Job drawing, mm, ordinate dimensions from the low corner. One solid piece. Coordinates: 2 decimals unless noted, no trailing zeros. Loops run counter-clockwise (first coordinate to the right, second up) from the corner with the lowest first, then second, coordinate; pieces in that order, holes last. Notation, with made-up numbers: (81.5, 1.25) - (132.5, 1.25) arc R10 ccw to (132.5, 10.25) - close; hole circle Ø6 at (-23.75, 8.25). An arc over 180 degrees is marked (long way). Use a Markdown table: item, result. Add a question column.
1. Band-saw the part on A-A, the plane y = 8.25. Give the cut face in (x, z).
2. Wall check: probe 1 along X at (y, z) = (1.75, 35); probe 2 along X at (y, z) = (4, 35.5) (1 decimal); probe 3 along Z at (x, y) = (50, 6). Give the ranges that are in metal, low to high. Write a range as [from, to].
3. Pull direction X, two halves, no side cores. Call the marked faces 1, 2, 3 and 4: pulls with the +X half, pulls with the -X half, needs draft (parallel to the pull), parting line crosses it, or undercut.
4. Band-saw the part on B-B, the plane x = 46.5. Give the cut face in (y, z), plus the area to 3 significant figures.
5. Band-saw the part on D-D, the plane y = 1.75. Give the cut face in (x, z).
6. Drop flat-ended pins along their axis: pin 1 (1 mm diameter, centred on x = 10.5, z = 52.5, fed in from -Y); pin 2 (6 mm diameter, centred on x = 11.5, y = 6.5, fed in from -Z); pin 3 (1 mm diameter, centred on y = 8, z = 56, fed in from +X). Give the stop position or say it passes through.
7. Band-saw the part on C-C, the plane z = 39. Give the cut face in (x, y) (1 decimal), plus the area to 3 significant figures.
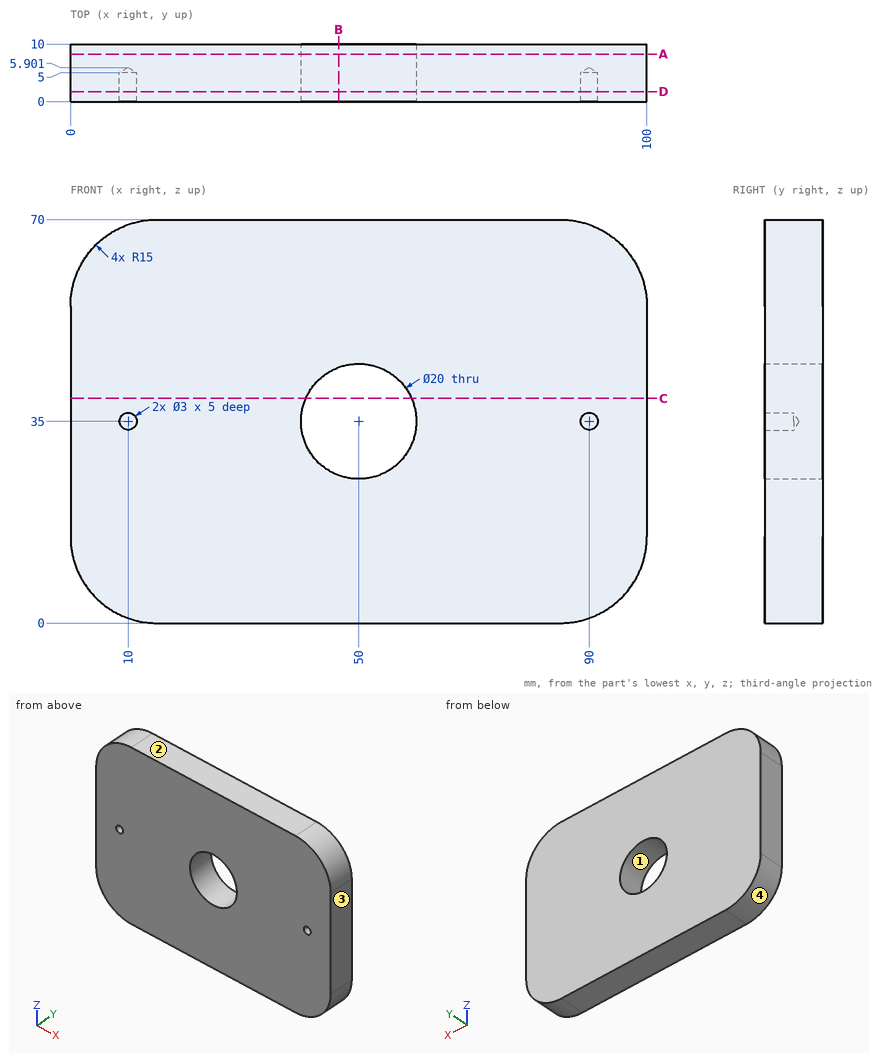
Geometry check:
| question | item | result |
|---|---|---|
| 1 | outline | (0, 15) arc R15 ccw to (15, 0) - (85, 0) arc R15 ccw to (100, 15) - (100, 55) arc R15 ccw to (85, 70) - (15, 70) arc R15 ccw to (0, 55) - close; hole circle Ø20 at (50, 35) |
| 2 | probe 1 | x = [0, 8.5], [11.5, 40], [60, 88.5], [91.5, 100] |
| 2 | probe 2 | x = [0, 8.6], [11.4, 40], [60, 88.6], [91.4, 100] |
| 2 | probe 3 | z = [0, 25], [45, 70] |
| 3 | face 1 | undercut |
| 3 | face 2 | needs draft |
| 3 | face 3 | pulls with the +X half |
| 3 | face 4 | pulls with the -X half |
| 4 | outline | (0, 0) - (10, 0) - (10, 25.63) - (0, 25.63) - close; (0, 44.37) - (10, 44.37) - (10, 70) - (0, 70) - close |
| 4 | area | 513 mm^2 |
| 5 | outline | (0, 15) arc R15 ccw to (15, 0) - (85, 0) arc R15 ccw to (100, 15) - (100, 55) arc R15 ccw to (85, 70) - (15, 70) arc R15 ccw to (0, 55) - close; hole circle Ø3 at (10, 35); hole circle Ø20 at (50, 35); hole circle Ø3 at (90, 35) |
| 6 | pin 1 | stops at y = 0 |
| 6 | pin 2 | stops at z = 0.01 |
| 6 | pin 3 | stops at x = 99.99 |
| 7 | outline | (0, 0) - (40.8, 0) - (40.8, 10) - (0, 10) - close; (59.2, 0) - (100, 0) - (100, 10) - (59.2, 10) - close |
| 7 | area | 817 mm^2 |
